from build123d import *

# Parameters (mm, degrees)
RESSALTO_EXTRUS_O1_DEPTH = 45
FILETE1_R                = 0.5
ESBO_O2_R                = 1.5
CORTE_EXTRUS_O1_DEPTH    = 46


with BuildPart() as part:
    # Esboço1 → Ressalto-extrusão1 (new body)
    with BuildSketch(Plane(origin=(0, 0, 0), x_dir=(-1, 0, 0), z_dir=(0, 0, -1))):
        Polygon((67.502122675, -1.443375673), (70.002122675, -2.886751346), (72.502122675, -1.443375673), (72.502122675, 1.443375673), (70.002122675, 2.886751346), (67.502122675, 1.443375673), align=None)
    extrude(amount=-RESSALTO_EXTRUS_O1_DEPTH)

    # Filete1
    filete1_edges = [part.edges().sort_by_distance(p)[0] for p in [
        (-71.252122675, -2.165063509, 45),
        (-72.502122675, 0, 45),
        (-71.252122675, 2.165063509, 45),
        (-68.752122675, 2.165063509, 45),
        (-67.502122675, 0, 45),
        (-68.752122675, 2.165063509, 0),
        (-71.252122675, 2.165063509, 0),
        (-72.502122675, 0, 0),
        (-71.252122675, -2.165063509, 0),
        (-68.752122675, -2.165063509, 0),
        (-67.502122675, 0, 0),
        (-68.752122675, -2.165063509, 45),
    ]]
    fillet(filete1_edges, radius=FILETE1_R)

    # Esboço2 → Corte-extrusão1 (cut, through all)
    with BuildSketch(Plane.XY.offset(45)):
        with Locations((-70.002122675, 0)):
            Circle(ESBO_O2_R)
    extrude(amount=-CORTE_EXTRUS_O1_DEPTH, mode=Mode.SUBTRACT)


solid = part.part
CAD build for the part. Positions are in the model's coordinates, mm. Round coordinates to 2 decimals unless told otherwise and drop trailing zeros. Loops run counter-clockwise (first coordinate to the right, second up) from the corner with the lowest first, then second, coordinate; pieces in that order, holes last. Notation, with made-up numbers: (62.5, 5.5) - (87.5, 5.5) arc R11 ccw to (87.5, 24.5) - close; hole circle Ø1 at (-10, 74). An arc over 180 degrees is marked (long way). Put each result on its own line as item: value.
1. Slice it at B-B on z = 39.5. List the corners of the cut face in (x, y).
Geometry check:
outline: (-72.5, -1.44) - (-70, -2.89) - (-67.5, -1.44) - (-67.5, 1.44) - (-70, 2.89) - (-72.5, 1.44) - close; hole circle Ø3 at (-70, 0)
2. Pin check, flat tip, straight feed: P1, Ø1.8, axis at x = -70, y = 0, coming from the -Z side. Stop position of the tip, or through.
Geometry check:
P1: through
3. Slice it at A-A on y = 0. List the corners of the cut face in (x, z), and give its area (3 significant figures).
Geometry check:
outline: (-72.5, 0.5) arc R0.5 ccw to (-72, 0) - (-71.5, 0) - (-71.5, 45) - (-72, 45) arc R0.5 ccw to (-72.5, 44.5) - close; (-68.5, 0) - (-68, 0) arc R0.5 ccw to (-67.5, 0.5) - (-67.5, 44.5) arc R0.5 ccw to (-68, 45) - (-68.5, 45) - close
area: 89.8 mm²
4. Wall check: line 1 (X direction, y = -0.05, z = 15); line 2 (X direction, y = -1, z = 33.5); line 3 (Y direction, x = -69.9, z = 10.5). Give the ranges that are in metal, low to high.
Geometry check:
line 1: -72.5 to -71.5, -68.5 to -67.5
line 2: -72.5 to -71.12, -68.88 to -67.5
line 3: -2.83 to -1.5, 1.5 to 2.83
5. Two-plate mould, pull along X, no slides. Class faces 1 (the cylindrical face through (-68.57, 0.45, 22.82)), 2 (the cylindrical face through (-71.16, 2.05, 0.15)), 3 (the flat face through (-67.502, 0, 22)): released by +X, released by -X, zero draft, split by the parting line, or undercut.
Geometry check:
face 1: undercut
face 2: released by -X
face 3: released by +X
